```python
from build123d import *

# Parameters (mm, degrees)
SKETCH1_W               = 55
SKETCH1_H               = 22
BOSS_EXTRUDE1_DEPTH     = 2
BOSS_EXTRUDE2_DEPTH     = 32.2
SKETCH5_R               = 1.3
CUT_EXTRUDE2_DEPTH      = 8
SKETCH1_2_W             = 55
SKETCH1_2_H             = 22
BOSS_EXTRUDE3_DEPTH     = 10
SKETCH11_R              = 1.5
CUT_EXTRUDE8_DEPTH      = 10
CUT_EXTRUDE9_DEPTH      = 5
CUT_EXTRUDE9_DEPTH_BACK = 46.242568451
SKETCH8_4_R             = 6.6
CUT_EXTRUDE10_DEPTH     = 10
SKETCH12_W              = 55
SKETCH12_H              = 44.2
BOSS_EXTRUDE4_DEPTH     = 1.5
FILLET1_R               = 6
CUT_EXTRUDE7_DEPTH      = 50.090630471
CUT_EXTRUDE7_DEPTH_BACK = 50.090630471
SKETCH10_W              = 12
SKETCH10_H              = 8


with BuildPart() as part:
    # Sketch1 → Boss-Extrude1 (new body)
    with BuildSketch(Plane(origin=(0, 0, 0), x_dir=(1, 0, 0), z_dir=(0, 1, 0))):
        Rectangle(SKETCH1_W, SKETCH1_H)
    extrude(amount=BOSS_EXTRUDE1_DEPTH)

    # Sketch2 → Boss-Extrude2 (add)
    with BuildSketch(Plane(origin=(0, 2, 0), x_dir=(1, 0, 0), z_dir=(0, 1, 0))):
        Polygon((-27.5, -11), (-27.5, 11), (27.5, 11), (27.5, -11), (20.5, -11), (20.5, 9.5), (-20.5, 9.5), (-20.5, -11), align=None)
    extrude(amount=BOSS_EXTRUDE2_DEPTH)

    # Sketch5 → Cut-Extrude2 (cut)
    with BuildSketch(Plane(origin=(0, 34.2, 0), x_dir=(1, 0, 0), z_dir=(0, 1, 0))):
        with Locations(Location((-24.75, -6, 0), (0, 0, 270))):
            Circle(SKETCH5_R)
        with Locations(Location((-24.75, 4, 0), (0, 0, 270))):
            Circle(SKETCH5_R)
        with Locations(Location((24.75, 4, 0), (0, 0, 270))):
            Circle(SKETCH5_R)
        with Locations(Location((24.75, -6, 0), (0, 0, 270))):
            Circle(SKETCH5_R)
    extrude(amount=-CUT_EXTRUDE2_DEPTH, mode=Mode.SUBTRACT)

    # Sketch1_2 → Boss-Extrude3 (add)
    with BuildSketch(Plane(origin=(0, 0, 0), x_dir=(1, 0, 0), z_dir=(0, 1, 0))):
        Rectangle(SKETCH1_2_W, SKETCH1_2_H)
    extrude(amount=-BOSS_EXTRUDE3_DEPTH)

    # Sketch11 → Cut-Extrude8 (cut)
    with BuildSketch(Plane.XZ.offset(10)):
        with Locations(Location((14.828145062, -4.942715021, 0), (0, 0, 270))):
            Circle(SKETCH11_R)
        with Locations(Location((14.828145062, 4.942715021, 0), (0, 0, 270))):
            Circle(SKETCH11_R)
        with Locations(Location((4.942715021, -4.942715021, 0), (0, 0, 270))):
            Circle(SKETCH11_R)
        with Locations(Location((4.942715021, 4.942715021, 0), (0, 0, 270))):
            Circle(SKETCH11_R)
        with Locations(Location((-4.942715021, -4.942715021, 0), (0, 0, 270))):
            Circle(SKETCH11_R)
        with Locations(Location((-4.942715021, 4.942715021, 0), (0, 0, 270))):
            Circle(SKETCH11_R)
        with Locations(Location((-14.828145062, -4.942715021, 0), (0, 0, 270))):
            Circle(SKETCH11_R)
        with Locations(Location((-14.828145062, 4.942715021, 0), (0, 0, 270))):
            Circle(SKETCH11_R)
    extrude(amount=-CUT_EXTRUDE8_DEPTH, mode=Mode.SUBTRACT)

    # Sketch8 → Cut-Extrude9 (cut, two sides: drawn at the far end of the back side and taken through both)
    with BuildSketch(Plane.XZ.offset(-CUT_EXTRUDE9_DEPTH_BACK)):
        with BuildLine():
            ThreePointArc((11, -3.2), (13.2627417, -2.2627417), (14.2, 0))
            Line((14.2, 0), (11, 0))
            Line((11, 0), (11, -3.2))
        make_face()
        with BuildLine():
            Line((11, 0), (14.2, 0))
            ThreePointArc((14.2, 0), (8.7372583, 2.2627417), (11, -3.2))
            Line((11, -3.2), (11, 0))
        make_face()
    extrude(amount=CUT_EXTRUDE9_DEPTH + CUT_EXTRUDE9_DEPTH_BACK, mode=Mode.SUBTRACT)

    # Sketch8_4 → Cut-Extrude10 (cut)
    with BuildSketch(Plane.XZ):
        with Locations(Location((11, 0, 0), (0, 0, 294.715710833))):
            Circle(SKETCH8_4_R)
    extrude(amount=-CUT_EXTRUDE10_DEPTH, mode=Mode.SUBTRACT)

    # Sketch12 → Boss-Extrude4 (add)
    with BuildSketch(Plane.XY.offset(11)):
        with Locations((0, 12.1)):
            Rectangle(SKETCH12_W, SKETCH12_H)
    extrude(amount=BOSS_EXTRUDE4_DEPTH)

    # Fillet1
    fillet1_edges = [part.edges().sort_by_distance(p)[0] for p in [
        (27.5, 12.1, 12.5),
        (-27.5, 12.1, 12.5),
        (-27.5, 12.1, -11),
        (27.5, 12.1, -11),
    ]]
    fillet(fillet1_edges, radius=FILLET1_R)

    # Sketch10 → Cut-Extrude7 (cut, two sides: drawn at the far end of the back side and taken through both)
    with BuildSketch(Plane.XY.offset(-9.5).offset(-CUT_EXTRUDE7_DEPTH_BACK)):
        with Locations((6, 10.5)):
            Rectangle(SKETCH10_W, SKETCH10_H)
    extrude(amount=CUT_EXTRUDE7_DEPTH + CUT_EXTRUDE7_DEPTH_BACK, mode=Mode.SUBTRACT)


solid = part.part
```
Geometry: final body of the model. Coordinates: model frame, mm. A direction names the side the tool comes from. Round coordinates to 2 decimals unless told otherwise and drop trailing zeros. Loops run counter-clockwise (first coordinate to the right, second up) from the corner with the lowest first, then second, coordinate; pieces in that order, holes last. Notation, with made-up numbers: (82.5, 19.25) -> (141.5, 19.25) arc R37 ccw to (141.5, 57.25) -> close; hole circle Ø8 at (79, 18.25). An arc over 180 degrees is marked (long way). Use one line per item in the form item = value.
Item 1: Contact query for flat-ended pins moving along their axis: pin 1 Ø0.9 at (x, z) = (-14.5, 4.5) entering from -Y; pin 2 Ø1.3 at (x, z) = (-25, -4.5) entering from +Y; pin 3 Ø5 at (x, z) = (-4.94, 4.94) entering from +Y. Output: stop coordinate, or through.
Evaluation:
pin_1 = 0
pin_2 = 26.2
pin_3 = 2
Item 2: Access query for faces 4 (the flat face through (6, 6.5, 12)), 5 (the cylindrical face through (-15.4, -5.07, -6.33)), 6 (the cylindrical face through (23.48, 30.26, -4.28)). Directions: +Z, -Z, +X, -X, +Y, -Y. A direction counts if a zero-diameter tool reaches every point of the face in a straight line with its end or side. Return the directions, or none.
Evaluation:
face_4 = +Z, -Z
face_5 = -Y
face_6 = +Y
Item 3: Material intervals for probe 1 along X at (y, z) = (28.75, 6); probe 2 along Z at (x, y) = (12, 32.5); probe 3 along Z at (x, y) = (11, -1.55), sorted ascending.
Evaluation:
probe_1 = -27.5 to -26.05, -23.45 to -20.5, 20.5 to 23.45, 26.05 to 27.5
probe_2 = -11 to -9.5, 11 to 12.5
probe_3 = -11 to -3.2, 3.2 to 12.5
Item 4: Cut plane C-C on x = -18. Output: boundary loops of the cut face in (y, z).
Evaluation:
outline = (-10, -11) -> (34.2, -11) -> (34.2, -9.5) -> (2, -9.5) -> (2, 11) -> (34.2, 11) -> (34.2, 12.5) -> (-10, 12.5) -> close
Item 5: Cut plane A-A on y = 16.5. Output: boundary loops of the cut face in (x, z).
Evaluation:
outline = (-27.5, -5) arc R6 ccw to (-21.5, -11) -> (21.5, -11) arc R6 ccw to (27.5, -5) -> (27.5, 6.5) arc R6 ccw to (21.5, 12.5) -> (-21.5, 12.5) arc R6 ccw to (-27.5, 6.5) -> close; hole (-20.5, -9.5) -> (20.5, -9.5) -> (20.5, 11) -> (-20.5, 11) -> close
Item 6: Draft query along Z for faces 1 (the cylindrical face through (-25.789, 12.409, 10.696)), 2 (the flat face through (0, 34.2, -10)), 3 (the cylindrical face through (4.368, -5.07, 3.557)). Return one class per face: released by +Z, released by -Z, zero draft, split by the parting line, or undercut.
Evaluation:
face_1 = released by +Z
face_2 = zero draft
face_3 = undercut
Item 7: Cut plane B-B on y = 11. Output: boundary loops of the cut face in (x, z).
Evaluation:
outline = (-27.5, -5) arc R6 ccw to (-21.5, -11) -> (0, -11) -> (0, -9.5) -> (-20.5, -9.5) -> (-20.5, 11) -> (0, 11) -> (0, 12.5) -> (-21.5, 12.5) arc R6 ccw to (-27.5, 6.5) -> close; (12, -11) -> (21.5, -11) arc R6 ccw to (27.5, -5) -> (27.5, 6.5) arc R6 ccw to (21.5, 12.5) -> (12, 12.5) -> (12, 11) -> (20.5, 11) -> (20.5, -9.5) -> (12, -9.5) -> close
Item 8: Cut plane D-D on y = -4. Give the number of separate pieces and of enclosed holes in the cut face, then the cut area to 3 significant figures.
Evaluation:
separate_pieces = 1
enclosed_holes = 9
area = 1,170 mm2
